For this review, take the finished solid that the model builds, in its own axes (mm). Face numbers are marked on the shaded views. Round coordinates to 2 decimals unless told otherwise and drop trailing zeros. Write each loop counter-clockwise with the first axis right and the second up, starting at its lowest first coordinate (ties: lowest second). Pieces come first, ordered by that corner, then holes.
from build123d import *

# Parameters (mm, degrees)
PAD_DEPTH    = 22.7
SKETCH001_W  = 8
SKETCH001_H  = 43.4
POCKET_DEPTH = 1.5
SKETCH002_R  = 0.5
PAD001_DEPTH = 1
SKETCH003_R  = 0.5
PAD002_DEPTH = 1


with BuildPart() as part:
    # Sketch → Pad (new body, symmetric)
    with BuildSketch(Plane.YZ):
        with BuildLine():
            Line((-6, 1.5), (6, 1.5))
            ThreePointArc((6, -1.5), (7.5, 0), (6, 1.5))
            Line((6, -1.5), (-6, -1.5))
            ThreePointArc((-6, 1.5), (-7.5, 0), (-6, -1.5))
        make_face()
    extrude(amount=PAD_DEPTH, both=True)

    # Sketch001 (on Face1 of Pad) → Pocket (cut)
    with BuildSketch(Plane.YX.offset(1.5)):
        Rectangle(SKETCH001_W, SKETCH001_H)
    extrude(amount=-POCKET_DEPTH, mode=Mode.SUBTRACT)

    # Sketch002 (on Face4 of Pocket) → Pad001 (join)
    with BuildSketch(Plane.YZ.offset(22.7)):
        with Locations((6, 0)):
            Circle(SKETCH002_R)
    extrude(amount=PAD001_DEPTH)

    # Sketch003 (on Face3 of Pad001) → Pad002 (join)
    with BuildSketch(Plane(origin=(-22.7, 0, 0), x_dir=(0, 1, 0), z_dir=(-1, 0, 0))):
        with Locations((6, 0)):
            Circle(SKETCH003_R)
    extrude(amount=PAD002_DEPTH)


solid = part.part
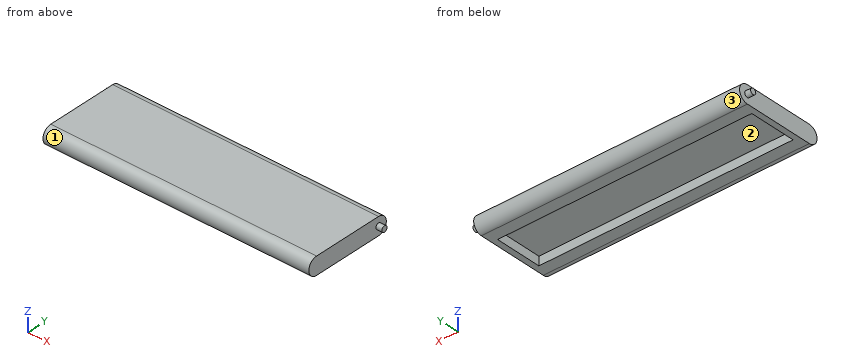
(1) For pin 1 Ø0.8 at (x, z) = (-10.5, -0.5) entering from +Y; pin 2 Ø1.2 at (y, z) = (1, -0.5) entering from -X; pin 3 Ø2.5 at (x, y) = (5.5, 1.5) entering from -Z, all flat-tipped, find the tip position at first contact; note any pin that passes through.
Geometry check:
pin 1: stops at y = 7.5
pin 2: stops at x = -22.7
pin 3: stops at z = 0
(2) Mouldability with a two-part tool opening along Y and no side actions: class the marked faces 1, 2 and 3 as pulls with the +Y half, pulls with the -Y half, needs draft (parallel to the pull), parting line crosses it, or undercut.
Geometry check:
face 1: pulls with the -Y half
face 2: undercut
face 3: pulls with the +Y half
(3) For line 1 along X through (y, z) = (-2, -0.05); line 2 along X through (y, z) = (3.5, 1.1); line 3 along Z through (x, y) = (0, -1.75), list the stretches that pass through material, from the lowest coordinate up.
Geometry check:
line 1: x = -22.7 to -21.7, 21.7 to 22.7
line 2: x = -22.7 to 22.7
line 3: z = 0 to 1.5
(4) We need section C-C, the plane z = -1.05. Give the boundary of the cut face in (x, y), and give its area (3 significant figures).
Geometry check:
outline: (-22.7, -7.07) - (22.7, -7.07) - (22.7, 7.07) - (-22.7, 7.07) - close; hole (-21.7, -4) - (21.7, -4) - (21.7, 4) - (-21.7, 4) - close
area: 295 mm2
(5) We need section A-A, the plane y = -3.25. Give the boundary of the cut face in (x, z), and give its area (3 significant figures).
Geometry check:
outline: (-22.7, -1.5) - (-21.7, -1.5) - (-21.7, 0) - (21.7, 0) - (21.7, -1.5) - (22.7, -1.5) - (22.7, 1.5) - (-22.7, 1.5) - close
area: 71.1 mm2
(6) We need section B-B, the plane x = 12. Give the boundary of the cut face in (y, z), and give its area (3 significant figures).
Geometry check:
outline: (-6, -1.5) - (-4, -1.5) - (-4, 0) - (4, 0) - (4, -1.5) - (6, -1.5) arc R1.5 ccw to (6, 1.5) - (-6, 1.5) arc R1.5 ccw to start
area: 31.1 mm2
